```python
from build123d import *

# Parameters (mm, degrees)
SKETCH2_W           = 114.3
SKETCH2_H           = 76.2
BOSS_EXTRUDE1_DEPTH = 152.4
SKETCH3_W           = 76.2
SKETCH3_H           = 38.1
CUT_EXTRUDE1_DEPTH  = 2.54
FILLET2_R           = 15.24
SKETCH4_W           = 40.64
SKETCH4_H           = 5.08
CUT_EXTRUDE2_DEPTH  = 20.32
SKETCH5_R           = 4.562719015
BOSS_EXTRUDE2_DEPTH = 2.54
SKETCH11_R          = 10.195906114
BOSS_EXTRUDE3_DEPTH = 2.54
SKETCH12_R          = 5.08
CUT_EXTRUDE8_DEPTH  = 15.24
SKETCH13_R          = 6.35
CUT_EXTRUDE9_DEPTH  = 15.24
FILLET3_R           = 2.54
FILLET4_R           = 2.54
BOSS_EXTRUDE4_DEPTH = 2.54
BOSS_EXTRUDE5_DEPTH = 2.54
SKETCH8_R           = 3.879636345
BOSS_EXTRUDE6_DEPTH = 2.54
BOSS_EXTRUDE7_DEPTH = 2.54
SKETCH9_R           = 8.218720736
BOSS_EXTRUDE8_DEPTH = 2.54


with BuildPart() as part:
    # Sketch2 → Boss-Extrude1 (new body)
    with BuildSketch(Plane(origin=(0, 0, 0), x_dir=(1, 0, 0), z_dir=(0, 1, 0))):
        Rectangle(SKETCH2_W, SKETCH2_H)
    extrude(amount=BOSS_EXTRUDE1_DEPTH)

    # Sketch3 → Cut-Extrude1 (cut)
    with BuildSketch(Plane.XY.offset(38.1)):
        with Locations((0, 120.65)):
            Rectangle(SKETCH3_W, SKETCH3_H)
    extrude(amount=-CUT_EXTRUDE1_DEPTH, mode=Mode.SUBTRACT)

    # Fillet2
    fillet2_edges = [part.edges().sort_by_distance(p)[0] for p in [
        (-57.15, 152.4, 0),
        (57.15, 152.4, 0),
        (-57.15, 0, 0),
        (57.15, 0, 0),
    ]]
    fillet(fillet2_edges, radius=FILLET2_R)

    # Sketch4 → Cut-Extrude2 (cut)
    with BuildSketch(Plane.XY.offset(38.1)):
        with Locations((-24.13, 78.74)):
            Rectangle(SKETCH4_W, SKETCH4_H)
    extrude(amount=-CUT_EXTRUDE2_DEPTH, mode=Mode.SUBTRACT)

    # Sketch5 → Boss-Extrude2 (add)
    with BuildSketch(Plane.XY.offset(38.1)):
        with Locations(Location((29.657673596, 81.713285476, 0), (0, 0, 180))):
            Circle(SKETCH5_R)
    extrude(amount=BOSS_EXTRUDE2_DEPTH)

    # Sketch11 → Boss-Extrude3 (add)
    with BuildSketch(Plane.ZY.offset(57.15)):
        with Locations(Location((0, 61.307792105, 0), (0, 0, 180))):
            Circle(SKETCH11_R)
    boss_extrude3 = extrude(amount=BOSS_EXTRUDE3_DEPTH)

    # Sketch12 → Cut-Extrude8 (cut)
    with BuildSketch(Plane.ZY.offset(59.69)):
        with Locations((0, 61.307792105)):
            Circle(SKETCH12_R)
    cut_extrude8 = extrude(amount=-CUT_EXTRUDE8_DEPTH, mode=Mode.SUBTRACT)

    # Mirror1: Boss-Extrude3, Cut-Extrude8 across plane
    add(boss_extrude3.mirror(Plane(origin=(0, 0, 0), x_dir=(0, 0, 1), z_dir=(1, 0, 0))))
    add(cut_extrude8.mirror(Plane(origin=(0, 0, 0), x_dir=(0, 0, 1), z_dir=(1, 0, 0))), mode=Mode.SUBTRACT)

    # Sketch13 → Cut-Extrude9 (cut)
    with BuildSketch(Plane.XZ):
        with Locations(Location((-25.4, 0, 0), (0, 0, 270))):
            Circle(SKETCH13_R)
        with Locations(Location((25.4, 0, 0), (0, 0, 270))):
            Circle(SKETCH13_R)
    extrude(amount=-CUT_EXTRUDE9_DEPTH, mode=Mode.SUBTRACT)

    # Fillet3
    fillet3_edges = [part.edges().sort_by_distance(p)[0] for p in [
        (-59.69, 61.307792105, 10.195906114),
        (59.69, 61.307792105, 10.195906114),
    ]]
    fillet(fillet3_edges, radius=FILLET3_R - 0.0001)  # a hair under: the kernel refuses the full size

    # Fillet4
    fillet4_edges = [part.edges().sort_by_distance(p)[0] for p in [
        (0, 101.6, 38.1),
        (-38.1, 120.65, 38.1),
        (38.1, 120.65, 38.1),
        (0, 139.7, 38.1),
    ]]
    fillet(fillet4_edges, radius=FILLET4_R - 0.0001)  # a hair under: the kernel refuses the full size

    # Sketch6 → Boss-Extrude4 (add)
    with BuildSketch(Plane.XY.offset(38.1)):
        Polygon((-34.29, 60.96), (-34.29, 55.88), (-39.37, 55.88), (-39.37, 50.8), (-34.29, 50.8), (-34.29, 45.72), (-29.21, 45.72), (-29.21, 50.8), (-24.13, 50.8), (-24.13, 55.88), (-29.21, 55.88), (-29.21, 60.96), align=None)
    extrude(amount=BOSS_EXTRUDE4_DEPTH)

    # Sketch7 → Boss-Extrude5 (add)
    with BuildSketch(Plane.XY.offset(38.1)):
        Polygon((17.617165085, 57.125299675), (13.181188265, 50.661447737), (22.053141905, 50.661447737), align=None)
    extrude(amount=BOSS_EXTRUDE5_DEPTH)

    # Sketch8 → Boss-Extrude6 (add)
    with BuildSketch(Plane.XY.offset(38.1)):
        with Locations(Location((31.558806519, 42.549947266, 0), (0, 0, 180))):
            Circle(SKETCH8_R)
    extrude(amount=BOSS_EXTRUDE6_DEPTH)

    # Sketch10 → Boss-Extrude7 (add)
    with BuildSketch(Plane.XY.offset(38.1)):
        with BuildLine():
            Line((-40.937728938, 31.776860704), (-33.713423831, 31.776860704))
            ThreePointArc((-33.713423831, 31.776860704), (-32.319259688, 30.38269656), (-33.713423831, 28.988532417))
            Line((-33.713423831, 28.988532417), (-40.937728938, 28.988532417))
            ThreePointArc((-40.937728938, 28.988532417), (-42.331893081, 30.38269656), (-40.937728938, 31.776860704))
        make_face()
        with BuildLine():
            Line((-23.827532632, 32.537313873), (-16.98345411, 32.537313873))
            ThreePointArc((-16.98345411, 32.537313873), (-14.828836798, 30.38269656), (-16.98345411, 28.228079248))
            Line((-16.98345411, 28.228079248), (-23.827532632, 28.228079248))
            ThreePointArc((-23.827532632, 28.228079248), (-25.982149945, 30.38269656), (-23.827532632, 32.537313873))
        make_face()
    extrude(amount=BOSS_EXTRUDE7_DEPTH)

    # Sketch9 → Boss-Extrude8 (add)
    with BuildSketch(Plane.XY.offset(38.1)):
        with Locations(Location((18.757844838, 33.677993627, 0), (0, 0, 180))):
            Circle(SKETCH9_R)
    extrude(amount=BOSS_EXTRUDE8_DEPTH)


solid = part.part
```
The listing builds one solid part. Answer for the finished solid, in the listing's coordinates (mm). A direction names the side the tool comes from. Round coordinates to 2 decimals unless told otherwise and drop trailing zeros. Loops run counter-clockwise (first coordinate to the right, second up) from the corner with the lowest first, then second, coordinate; pieces in that order, holes last.
Q1. Given pin 1 Ø1.3 at (y, z) = (58, 40) entering from -X; pin 2 Ø1 at (y, z) = (61, 30.5) entering from -X; pin 3 Ø0.8 at (x, z) = (-38.5, 39.5) entering from +Y, each flat-ended and moving along its own axis, determine where each tip first touches the part or whether it passes through.
Q2. Section B-B, the plane z = 22.5 is taken. Determine the outline of the cut face in (x, y), then the cut area to 3 significant figures.
Q3. Find the intervals of material crossed by line 1 (Z direction, x = -25, y = 9); line 2 (X direction, y = 81, z = 27); line 3 (Y direction, x = -11, z = 20), in increasing order.
Q4. Section D-D, the plane z = -16 is taken. Determine the outline of the cut face in (x, y), then the cut area to 3 significant figures.
Q5. Which of the six approach directions +Z, -Z, +X, -X, +Y, -Y give full straight-line access (tool end or side, diameter ignored) to faces 4 (the face through (-24, 81.28, 28)), 5 (the face through (-44.45, 61, 0)), 6 (the face through (15.43, 53.94, 39.35)), 7 (the face through (19.766, 7.513, -2.93)), 8 (the face through (44.45, 61, 0))?
Q6. For a pull along X with two mould halves and no side action, classify faces 1 (the face through (29.769, 45.992, 39.352)), 2 (the face through (19.9, 53.8, 39.4)), 3 (the face through (-59.69, 66.3, -1.6)) as released by +X, released by -X, zero draft, split by the parting line, or undercut.
Completed:
1. pin 1: stops at x = -34.29
1. pin 2: stops at x = -57.15
1. pin 3: stops at y = 55.88
2. outline: (-57.15, 15.24) arc R15.24 ccw to (-41.91, 0) - (41.91, 0) arc R15.24 ccw to (57.15, 15.24) - (57.15, 137.16) arc R15.24 ccw to (41.91, 152.4) - (-41.91, 152.4) arc R15.24 ccw to (-57.15, 137.16) - close; hole (-44.45, 76.2) - (-3.81, 76.2) - (-3.81, 81.28) - (-44.45, 81.28) - close
2. area: 17,000 mm2
3. line 1: z = -38.1 to -6.34, 6.34 to 38.1
3. line 2: x = -57.15 to -44.45, -3.81 to 57.15
3. line 3: y = 0 to 76.2, 81.28 to 152.4
4. outline: (-57.15, 15.24) arc R15.24 ccw to (-41.91, 0) - (41.91, 0) arc R15.24 ccw to (57.15, 15.24) - (57.15, 137.16) arc R15.24 ccw to (41.91, 152.4) - (-41.91, 152.4) arc R15.24 ccw to (-57.15, 137.16) - close
4. area: 17,200 mm2
5. face 4: +Z
5. face 5: -X
5. face 6: +Z, +Y
5. face 7: -Y
5. face 8: +X
6. face 1: undercut
6. face 2: released by +X
6. face 3: released by -X
